```python
from build123d import *

# Parameters (mm, degrees)
SKETCH1_R           = 3.048
BOSS_EXTRUDE1_DEPTH = 1.905
CUT_EXTRUDE2_DEPTH  = 1.651
BOSS_EXTRUDE3_DEPTH = 1.27


with BuildPart() as part:
    # Sketch1 → Boss-Extrude1 (new body)
    with BuildSketch(Plane.XY):
        with BuildLine():
            Line((-13.231934716, 13.729837747), (-15.263934716, 31.509837747))
            ThreePointArc((-15.263934716, 31.509837747), (-21.261976505, 33.200417113), (-22.702706225, 27.137508425))
            ThreePointArc((-22.702706225, 27.137508425), (-21.220829792, 20.52075151), (-21.455464715, 13.744146439))
            ThreePointArc((-21.455464715, 13.744146439), (-22.988481312, -1.727276666), (-22.555391654, -17.268431904))
            ThreePointArc((-22.555391654, -17.268431904), (-20.128095916, -16.969854608), (-18.819934716, -19.036162253))
            Line((-18.819934716, -19.036162253), (-17.534121248, -22.084162253))
            ThreePointArc((-17.534121248, -22.084162253), (-18.691312873, -25.205533652), (-21.737196185, -23.862162253))
            Line((-21.737196185, -23.862162253), (-19.581934716, -31.990162253))
            ThreePointArc((-19.581934716, -31.990162253), (-15.392244863, -32.759368057), (-11.199934716, -33.514162253))
            ThreePointArc((-11.199934716, -33.514162253), (-9.63879843, -32.898087249), (-8.919111875, -31.38192559))
            Line((-8.919111875, -31.38192559), (-8.355134716, -18.401162253))
            Line((-8.355134716, -18.401162253), (-12.063534716, -15.988162253))
            Line((-12.063534716, -15.988162253), (-12.825534716, -8.037962253))
            Line((-12.825534716, -8.037962253), (-9.777534716, -3.796162253))
            Line((-9.777534716, -3.796162253), (-10.945934716, 11.443837747))
            Line((-10.945934716, 11.443837747), (-13.231934716, 13.729837747))
        make_face()
        with Locations((-19.073934716, 29.477837747)):
            Circle(SKETCH1_R, mode=Mode.SUBTRACT)
        with Locations((-12.317534716, -28.103962253)):
            Circle(SKETCH1_R, mode=Mode.SUBTRACT)
    extrude(amount=BOSS_EXTRUDE1_DEPTH)

    # Sketch7 → Cut-Extrude2 (cut)
    with BuildSketch(Plane.XY):
        with BuildLine():
            Line((-10.945934716, 11.443837747), (-13.231934716, 13.729837747))
            ThreePointArc((-13.231934716, 13.729837747), (-14.796876411, 3.164765256), (-16.025932156, -7.444627811))
            ThreePointArc((-16.025932156, -7.444627811), (-14.913011554, -14.738413577), (-11.669461291, -21.365425329))
            ThreePointArc((-11.669461291, -21.365425329), (-10.207206492, -22.532020863), (-8.57425285, -23.444488198))
            Line((-8.57425285, -23.444488198), (-8.486546668, -21.42580149))
            ThreePointArc((-8.486546668, -21.42580149), (-11.247875767, -18.756621385), (-12.886743333, -15.283355784))
            ThreePointArc((-12.886743333, -15.283355784), (-13.652704618, -9.554942708), (-13.628126313, -3.775599409))
            ThreePointArc((-13.628126313, -3.775599409), (-12.336996698, 3.84292494), (-10.945934716, 11.443837747))
        make_face()
    extrude(amount=CUT_EXTRUDE2_DEPTH, mode=Mode.SUBTRACT)

    # Sketch8 → Boss-Extrude3 (add)
    with BuildSketch(Plane(origin=(0, 0, 0), x_dir=(-1, 0, 0), z_dir=(0, 0, -1))):
        with BuildLine():
            Line((8.355134716, -18.401162253), (8.486546668, -21.42580149))
            ThreePointArc((8.486546668, -21.42580149), (11.247875767, -18.756621385), (12.886743333, -15.283355784))
            ThreePointArc((12.886743333, -15.283355784), (13.652704618, -9.554942708), (13.628126313, -3.775599409))
            ThreePointArc((13.628126313, -3.775599409), (12.336996698, 3.84292494), (10.945934716, 11.443837747))
            Line((10.945934716, 11.443837747), (9.777534716, -3.796162253))
            Line((9.777534716, -3.796162253), (12.825534716, -8.037962253))
            Line((12.825534716, -8.037962253), (12.063534716, -15.988162253))
            Line((12.063534716, -15.988162253), (8.355134716, -18.401162253))
        make_face()
    extrude(amount=BOSS_EXTRUDE3_DEPTH)


solid = part.part
```
Check sheet for the modelled part. Datum: model origin and axes. Units: mm. A direction names the side the tool comes from. Coordinates: 2 decimals unless noted, no trailing zeros. Write each loop counter-clockwise with the first axis right and the second up, starting at its lowest first coordinate (ties: lowest second). Pieces come first, ordered by that corner, then holes. Notation, with made-up numbers: M 23,17 L 41,17 A36 cw 41,55 Z; hole C 55.25,-29 d6. An arc over 180 degrees is marked long. Write item = value, one per line. Start each with the question number.
1. Tool access check on faces 4 (the cylindrical face through (-13.647, -9.636, 0.211)), 5 (the cylindrical face through (-20.161, -16.955, 0.939)), 6 (the flat face through (-11.28, -5.89, 0.34)). Record the directions out of +Z, -Z, +X, -X, +Y, -Y that give a thin tool (end or side, any length) a straight path to the whole face; none if there is none.
2. Go/stop test with flat-tipped pins: pin 1 (8 mm diameter, centred on x = -15.5, y = 25.5, fed in from -Z); pin 2 (5.5 mm diameter, centred on x = -12.32, y = -28.1, fed in from -Z). Record where each tip stops, or that it passes through.
3. Mould release check, pull along Y, two halves, no side actions. Record for faces 1 (the flat face through (-20.675, -27.869, 0.939)), 2 (the flat face through (-16, 1, 1.905)), 3 (the flat face through (-14, -6, 1.651)): pulls with the +Y half, pulls with the -Y half, needs draft (parallel to the pull), parting line crosses it, or undercut.
4. Sectioned sample at D-D (y = 20). Record the cut outline in (x, z) (3 decimals), then the cut area to 3 significant figures.
5. Sectioned sample at A-A (z = 0.6). Record the cut outline in (x, y), then the cut area to 3 significant figures.
6. Sectioned sample at C-C (y = -2.5). Record the cut outline in (x, z) (3 decimals).
7. Thickness scan on probe 1 along Y at (x, z) = (-19.25, 0.8); probe 2 along Z at (x, y) = (-19.25, -13.5) (3 decimals); probe 3 along Z at (x, y) = (-15.75, -5.5) (3 decimals). Record the ranges inside material, lowest first.
8. Sectioned sample at B-B (y = 9.5). Record the cut outline in (x, z) (1 decimal), then the cut area to 3 significant figures.
The answers:
q1.face_4 = -Z
q1.face_5 = +Z, -Z
q1.face_6 = +Z, -Z, +X
q2.pin_1 = 0
q2.pin_2 = through
q3.face_1 = pulls with the -Y half
q3.face_2 = needs draft
q3.face_3 = undercut
q4.outline = M -21.177,0 L -13.949,0 L -13.949,1.905 L -21.177,1.905 Z
q4.area = 13.8 mm²
q5.outline = M -22.7,27.14 A26.67 cw -21.46,13.74 A122.86 ccw -22.56,-17.27 A2.29 cw -18.82,-19.04 L -17.53,-22.08 A2.29 cw long -21.74,-23.86 L -19.58,-31.99 A1238.76 ccw -11.2,-33.51 A2.29 ccw -8.92,-31.38 L -8.57,-23.44 A11.43 cw -11.67,-21.37 A24.38 cw -16.03,-7.44 A336.69 cw -13.23,13.73 L -15.26,31.51 A4.32 ccw long Z; M -13.63,-3.78 A42.16 ccw -12.89,-15.28 A10.68 ccw -8.49,-21.43 L -8.36,-18.4 L -12.06,-15.99 L -12.83,-8.04 L -9.78,-3.8 L -10.95,11.44 A588.43 ccw Z; hole C -19.07,29.48 d6.1; hole C -12.32,-28.1 d6.1
q5.area = 529 mm²
q6.outline = M -23.013,0 L -15.496,0 L -15.496,1.651 L -13.419,1.651 L -13.419,-1.27 L -9.877,-1.27 L -9.877,1.905 L -23.013,1.905 Z
q7.probe_1 = -32.05 to -25.36, -17.7 to 26.43, 32.52 to 33.79
q7.probe_2 = 0 to 1.905
q7.probe_3 = 1.651 to 1.905
q8.outline = M -22.1,0 L -13.9,0 L -13.9,1.7 L -11.3,1.7 L -11.3,-1.3 L -10.8,-1.3 L -10.8,1.9 L -22.1,1.9 Z
q8.area = 17.9 mm²
